Build history of the part. All positions in model axes, mm. Coordinates: 2 decimals unless noted, no trailing zeros. Write each loop counter-clockwise with the first axis right and the second up, starting at its lowest first coordinate (ties: lowest second). Pieces come first, ordered by that corner, then holes.
```python
from build123d import *

# Parameters (mm, degrees)
F0_W     = 45
F0_H     = 50
F1_DEPTH = 215
F2_SIZE  = 5
F3_R     = 10
F5_DEPTH = 45.001


with BuildPart() as f1:
    # F0 (on Front) → F1 (new body)
    with BuildSketch(Plane.XZ):
        Rectangle(F0_W, F0_H)
    extrude(amount=F1_DEPTH)

    # F2
    f2_edges = [f1.edges().sort_by_distance(p)[0] for p in [
        (22.5, -107.5, 25),
        (-22.5, -107.5, 25),
        (22.5, -107.5, -25),
        (-22.5, -107.5, -25),
        (22.5, -215, 0),
        (22.5, 0, 0),
        (-22.5, 0, 0),
    ]]
    chamfer(f2_edges, length=F2_SIZE)

    # F3
    f3_edges = [f1.edges().sort_by_distance(p)[0] for p in [
        (0, -215, 25),
        (0, -215, -25),
        (0, 0, 25),
        (0, 0, -25),
    ]]
    fillet(f3_edges, radius=F3_R)

    # F4 (on face) → F5 (cut, through all)
    with BuildSketch(Plane.YZ.offset(22.5)):
        with BuildLine():
            ThreePointArc((-210, 8.56e-08), (-195.0000000428, -15), (-180, 0))
            ThreePointArc((-180, 0), (-194.9999999572, 15), (-210, 8.56e-08))
        make_face()
    extrude(amount=-F5_DEPTH, mode=Mode.SUBTRACT)


solid = f1.part
```
1. Saw through at B-B on x = 14.5. List the corners of the cut face in (y, z).
Computed values:
outline: (-215, -15) arc R10 ccw to (-205, -25) - (-10, -25) arc R10 ccw to (0, -15) - (0, 15) arc R10 ccw to (-10, 25) - (-205, 25) arc R10 ccw to (-215, 15) - close; hole circle Ø30 at (-195, 0)
2. Saw through at D-D on y = -89.5. List the corners of the cut face in (x, z), plus the area to 3 significant figures.
Computed values:
outline: (-22.5, -20) - (-17.5, -25) - (17.5, -25) - (22.5, -20) - (22.5, 20) - (17.5, 25) - (-17.5, 25) - (-22.5, 20) - close
area: 2,200 mm2
3. Saw through at C-C on z = -4. List the corners of the cut face in (x, y).
Computed values:
outline: (-22.5, -215) - (17.5, -215) - (22.5, -210) - (22.5, -209.46) - (-22.5, -209.46) - close; (-22.5, -180.54) - (22.5, -180.54) - (22.5, -5) - (17.5, 0) - (-17.5, 0) - (-22.5, -5) - close
4. Saw through at A-A on y = -195. List the corners of the cut face in (x, z), plus the area to 3 significant figures.
Computed values:
outline: (-22.5, -20) - (-17.5, -25) - (17.5, -25) - (22.5, -20) - (22.5, -15) - (-22.5, -15) - close; (-22.5, 15) - (22.5, 15) - (22.5, 20) - (17.5, 25) - (-17.5, 25) - (-22.5, 20) - close
area: 850 mm2
5. Probe line 1 along Z through (x, y) = (2, -195); line 2 along Y through (x, z) = (-7, 0); line 3 along Y through (x, z) = (-3, -3). List the from-to ranges inside material, lowest first.
Computed values:
line 1: z = -25 to -15, 15 to 25
line 2: y = -215 to -210, -180 to 0
line 3: y = -215 to -209.7, -180.3 to 0
6. Mould opens along Y. For faces 1 (the face through (20, -2.5, -0.3)), 2 (the face through (-3, -215, 0)), 3 (the face through (0.315, -209.985, 0.66)), 4 (the face through (0, -106, 25)) say: +Y half, -Y half, draft (parallel to the pull), parting line (faces both ways), or undercut.
Computed values:
face 1: +Y half
face 2: -Y half
face 3: undercut
face 4: draft
